Study the drawing (mm; zero at the part's minimum x, y, z) and answer. A direction names the side the tool comes from. Give positions to 0.01 mm unless a question says otherwise; leave off trailing zeros. Write each loop counter-clockwise with the first axis right and the second up, starting at its lowest first coordinate (ties: lowest second). Pieces come first, ordered by that corner, then holes. Notation, with made-up numbers: (40.5, 13) - (97.5, 13) arc R16 ccw to (97.5, 30) - close; hole circle Ø2 at (-26, 2.5). An arc over 180 degrees is marked (long way). Return JSON: item names as keys, results as strings.
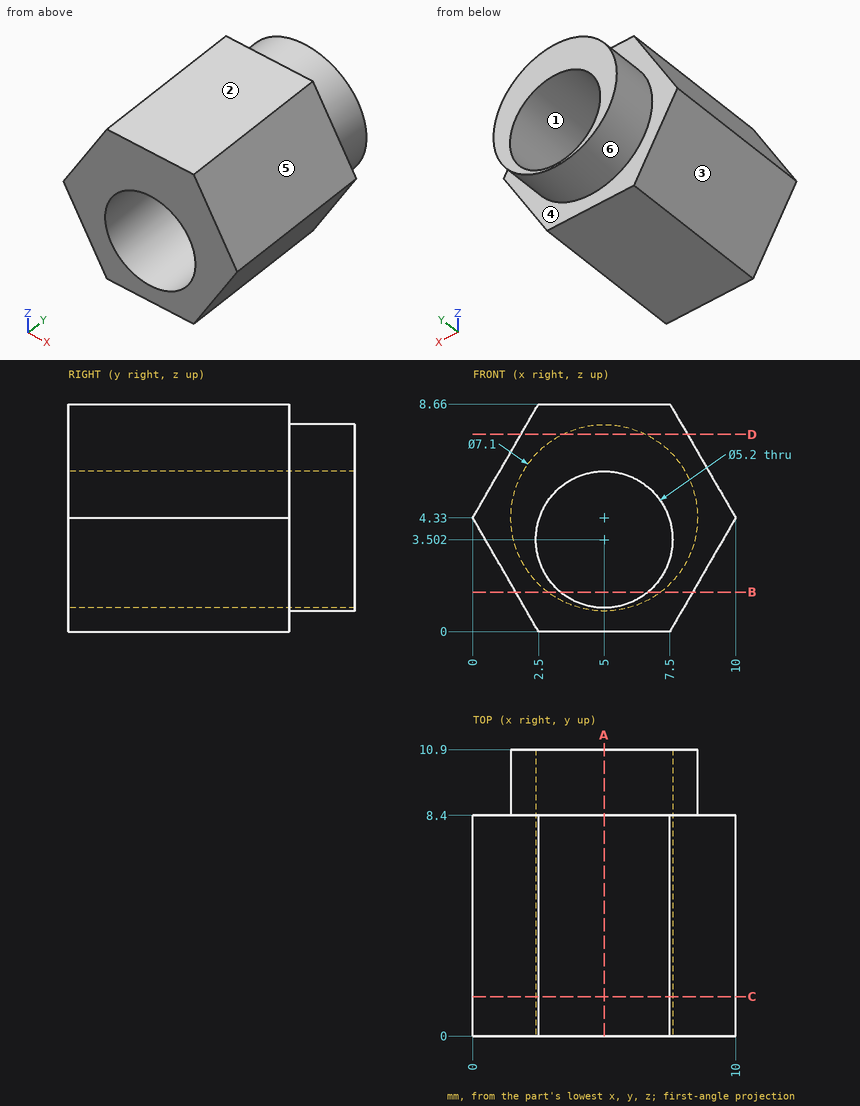
Item 1: Consider L1, parallel to Z at x = 5, y = 4.25; L2, parallel to Y at x = 3.75, z = 8.25; L3, parallel to X at y = 9.5, z = 2. Determine where each line is inside the solid, lowest interval first.
Answer below:
{"L1": "z = 0 to 0.9, 6.1 to 8.66", "L2": "y = 0 to 8.4", "L3": "x = 2.32 to 2.88, 7.12 to 7.68"}
Item 2: For the marked faces 5 and 6, determine the directions among +Z, -Z, +X, -X, +Y, -Y from which every point of the face is accessible in a straight line to the end or side of a thin tool.
Answer below:
{"face 5": "+Z, +X, +Y, -Y", "face 6": "+Y"}
Item 3: A cutting plane is placed at B-B on z = 1.5. Determine the outline of the cut face in (x, y), then the cut area to 3 significant figures.
Answer below:
{"outline": "(1.63, 0) - (3.34, 0) - (3.34, 10.9) - (2.86, 10.9) - (2.86, 8.4) - (1.63, 8.4) - close; (6.66, 0) - (8.37, 0) - (8.37, 8.4) - (7.14, 8.4) - (7.14, 10.9) - (6.66, 10.9) - close", "area": "31.1 mm²"}
Item 4: Flat-ended cylindrical pins translate along their axes: P1, Ø1, axis at x = 4.5, z = 3, coming from the +Y side; P2, Ø5, axis at y = 3.5, z = 1.5, coming from the -X side. Find the tip coordinate at first contact, or state that the pin passes through.
Answer below:
{"P1": "passes through", "P2": "stops at x = 0.19"}
Item 5: A cutting plane is placed at C-C on y = 1.5. Determine the outline of the cut face in (x, z), then the cut area to 3 significant figures.
Answer below:
{"outline": "(0, 4.33) - (2.5, 0) - (7.5, 0) - (10, 4.33) - (7.5, 8.66) - (2.5, 8.66) - close; hole circle Ø5.2 at (5, 3.5)", "area": "43.7 mm²"}
Item 6: The mould has two halves that part along Z. Classify the marked faces 1, 2, 3 and 4: +Z half, -Z half, draft (parallel to the pull), parting line (faces both ways), or undercut.
Answer below:
{"face 1": "undercut", "face 2": "+Z half", "face 3": "-Z half", "face 4": "draft"}
Item 7: A cutting plane is placed at A-A on x = 5. Determine the outline of the cut face in (y, z).
Answer below:
{"outline": "(0, 0) - (8.4, 0) - (8.4, 0.78) - (10.9, 0.78) - (10.9, 0.9) - (0, 0.9) - close; (0, 6.1) - (10.9, 6.1) - (10.9, 7.88) - (8.4, 7.88) - (8.4, 8.66) - (0, 8.66) - close"}
Item 8: A cutting plane is placed at D-D on z = 7.5. Determine the outline of the cut face in (x, y).
Answer below:
{"outline": "(1.83, 0) - (8.17, 0) - (8.17, 8.4) - (6.6, 8.4) - (6.6, 10.9) - (3.4, 10.9) - (3.4, 8.4) - (1.83, 8.4) - close"}
